The model under review builds one solid part; all positions refer to its coordinate system, in mm. A direction names the side the tool comes from. Give positions to 0.01 mm unless a question says otherwise; leave off trailing zeros. Loops run counter-clockwise (first coordinate to the right, second up) from the corner with the lowest first, then second, coordinate; pieces in that order, holes last. Notation, with made-up numbers: (44.25, 78.25) - (87.25, 78.25) arc R31 ccw to (87.25, 117.25) - close; hole circle Ø3 at (75, 56). An arc over 180 degrees is marked (long way). Answer as a JSON object with one key per item and string values.
from build123d import *

# Parameters (mm, degrees)
SKETCH1_W                      = 100
SKETCH1_H                      = 100
SKETCH1_W_2                    = 94
SKETCH1_H_2                    = 94
EXTRUDE_THIN1_DEPTH            = 130
FILLET1_R                      = 0.5
FILLET2_R                      = 3
F_8_0_8_DIAMETER_HOLE2_D       = 8
F_8_0_8_DIAMETER_HOLE3_D       = 8
F_10_0_10_DIAMETER_HOLE1_D     = 10
F_10_0_10_DIAMETER_HOLE2_D     = 10
M8X1_25_TAPPED_HOLE1_D         = 6.8
M8X1_25_TAPPED_HOLE1_DEPTH     = 3
M8X1_25_TAPPED_HOLE2_D         = 6.8
M8X1_25_TAPPED_HOLE2_DEPTH     = 3
F_21_0_21_DIAMETER_HOLE1_D     = 21
F_21_0_21_DIAMETER_HOLE1_DEPTH = 3
F_6_0_6_DIAMETER_HOLE1_D       = 6
F_6_0_6_DIAMETER_HOLE1_DEPTH   = 3
F_10_0_10_DIAMETER_HOLE4_D     = 10
F_10_0_10_DIAMETER_HOLE4_DEPTH = 3
SKETCH33_R                     = 4
CUT_EXTRUDE1_DEPTH             = 10


with BuildPart() as part:
    # Sketch1 → Extrude-Thin1 (new body)
    with BuildSketch(Plane.XY):
        Rectangle(SKETCH1_W, SKETCH1_H)
        Rectangle(SKETCH1_W_2, SKETCH1_H_2, mode=Mode.SUBTRACT)
    extrude(amount=EXTRUDE_THIN1_DEPTH)

    # Fillet1
    fillet1_edges = [part.edges().sort_by_distance(p)[0] for p in [
        (47, -47, 65),
        (47, 47, 65),
        (-47, 47, 65),
        (-47, -47, 65),
    ]]
    fillet(fillet1_edges, radius=FILLET1_R)

    # Fillet2
    fillet2_edges = [part.edges().sort_by_distance(p)[0] for p in [
        (50, -50, 65),
        (-50, -50, 65),
        (-50, 50, 65),
        (50, 50, 65),
    ]]
    fillet(fillet2_edges, radius=FILLET2_R)

    # Ø8.0 (8) Diameter Hole2 (through all)
    with Locations(Plane(origin=(0, 50, 0), x_dir=(1, 0, 0), z_dir=(0, 1, 0))):
        with Locations((28, -32), (28, -90)):
            Hole(F_8_0_8_DIAMETER_HOLE2_D / 2)

    # Ø8.0 (8) Diameter Hole3 (through all)
    with Locations(Plane(origin=(50, 0, 0), x_dir=(0, 0, -1), z_dir=(1, 0, 0))):
        with Locations((-14, 31), (-110, 31)):
            Hole(F_8_0_8_DIAMETER_HOLE3_D / 2)

    # Ø10.0 (10) Diameter Hole1 (through all)
    with Locations(Plane(origin=(0, 50, 0), x_dir=(1, 0, 0), z_dir=(0, 1, 0))):
        with Locations((-34, -56)):
            Hole(F_10_0_10_DIAMETER_HOLE1_D / 2)

    # Ø10.0 (10) Diameter Hole2 (through all)
    with Locations(Plane(origin=(50, 0, 0), x_dir=(0, 0, -1), z_dir=(1, 0, 0))):
        with Locations((-44, -31)):
            Hole(F_10_0_10_DIAMETER_HOLE2_D / 2)

    # M8x1.25 Tapped Hole1
    with Locations(Plane.ZY.offset(50)):
        with Locations((56, -15), (56, 35)):
            Hole(M8X1_25_TAPPED_HOLE1_D / 2, depth=M8X1_25_TAPPED_HOLE1_DEPTH)

    # M8x1.25 Tapped Hole2
    with Locations(Plane(origin=(0, -50, 0), x_dir=(-1, 0, 0), z_dir=(0, -1, 0))):
        with Locations((20, -44), (-35, -44)):
            Hole(M8X1_25_TAPPED_HOLE2_D / 2, depth=M8X1_25_TAPPED_HOLE2_DEPTH)

    # Ø21.0 (21) Diameter Hole1
    with Locations(Plane(origin=(50, 0, 0), x_dir=(0, 0, -1), z_dir=(1, 0, 0))):
        with Locations((-70, 0)):
            Hole(F_21_0_21_DIAMETER_HOLE1_D / 2, depth=F_21_0_21_DIAMETER_HOLE1_DEPTH)

    # Ø6.0 (6) Diameter Hole1
    with Locations(Plane(origin=(50, 0, 0), x_dir=(0, 0, -1), z_dir=(1, 0, 0))):
        with Locations((-41.157258279, -16.652364697), (-53.347635303, 28.842741721), (-98.842741721, 16.652364697), (-86.652364697, -28.842741721)):
            Hole(F_6_0_6_DIAMETER_HOLE1_D / 2, depth=F_6_0_6_DIAMETER_HOLE1_DEPTH)

    # Ø10.0 (10) Diameter Hole4
    with Locations(Plane(origin=(0, 50, 0), x_dir=(1, 0, 0), z_dir=(0, 1, 0))):
        with Locations((-3, -105)):
            Hole(F_10_0_10_DIAMETER_HOLE4_D / 2, depth=F_10_0_10_DIAMETER_HOLE4_DEPTH)

    # Sketch33 → Cut-Extrude1 (cut)
    with BuildSketch(Plane(origin=(0, 50, 0), x_dir=(1, 0, 0), z_dir=(0, 1, 0))):
        with Locations(Location((-33, -105, 0), (0, 0, 270))):
            Circle(SKETCH33_R)
    extrude(amount=-CUT_EXTRUDE1_DEPTH, mode=Mode.SUBTRACT)


solid = part.part
Q1. Consider section B-B, the plane z = 23. State the section outline as (x, y) points, plus the area to 3 significant figures.
Results:
{"outline": "(-50, -47) arc R3 ccw to (-47, -50) - (47, -50) arc R3 ccw to (50, -47) - (50, 47) arc R3 ccw to (47, 50) - (-47, 50) arc R3 ccw to (-50, 47) - close; hole (-47, -46.5) arc R0.5 ccw to (-46.5, -47) - (46.5, -47) arc R0.5 ccw to (47, -46.5) - (47, 46.5) arc R0.5 ccw to (46.5, 47) - (-46.5, 47) arc R0.5 ccw to (-47, 46.5) - close", "area": "1,160 mm^2"}
Q2. For faces 1 (the face through (48.479, 17.553, 101.704)), 2 (the face through (-48.48, 33.7, 52.86)), 3 (the face through (47, -11, 64)), 4 (the face through (-1.92, 48.48, 109.88)), list the 3-axis set-ups (+Z, -Z, +X, -X, +Y, -Y) from which the entire face can be reached by the end or side of a thin tool; tool diameter is ignored.
Results:
{"face 1": "+X", "face 2": "-X", "face 3": "+Z, -Z", "face 4": "+Y"}
Q3. Consider section A-A, the plane y = 41.5. State the section outline as (x, z) points.
Results:
{"outline": "(-50, 0) - (-47, 0) - (-47, 130) - (-50, 130) - close; (47, 0) - (50, 0) - (50, 130) - (47, 130) - close"}
Q4. To check wall thickness, follow probe 1 along Y at (x, z) = (17, 72); probe 2 along X at (y, z) = (49, 105). State the ranges of each line that lie inside material, in increasing order. Write a range as [from, to].
Results:
{"probe 1": "y = [-50, -47], [47, 50]", "probe 2": "x = [-49.24, -37], [-29, -8], [2, 49.24]"}
Q5. The part is to be moulded in two halves that separate along Z. For faces 5 (the face through (48.48, 0.46, 59.51)), 6 (the face through (-47, -1, 64)), say which applies: +Z half, -Z half, draft (parallel to the pull), parting line (faces both ways), or undercut.
Results:
{"face 5": "undercut", "face 6": "draft"}
Q6. Consider section D-D, the plane x = 28. State the section outline as (y, z) points.
Results:
{"outline": "(-50, 0) - (-47, 0) - (-47, 28) - (-50, 28) - close; (-50, 36) - (-47, 36) - (-47, 86) - (-50, 86) - close; (-50, 94) - (-47, 94) - (-47, 130) - (-50, 130) - close; (47, 0) - (50, 0) - (50, 28) - (47, 28) - close; (47, 36) - (50, 36) - (50, 86) - (47, 86) - close; (47, 94) - (50, 94) - (50, 130) - (47, 130) - close"}
